Part model, mm, in its own coordinate system. Face numbers are marked on the shaded views. Round coordinates to 2 decimals unless told otherwise and drop trailing zeros. Loops run counter-clockwise (first coordinate to the right, second up) from the corner with the lowest first, then second, coordinate; pieces in that order, holes last. Notation, with made-up numbers: (-5.5, -4) -> (43.5, -4) arc R23 cw to (43.5, 7) -> close; hole circle Ø11 at (13, 15.25). An arc over 180 degrees is marked (long way). Answer as a JSON object with one key per item and string values. Group by question number.
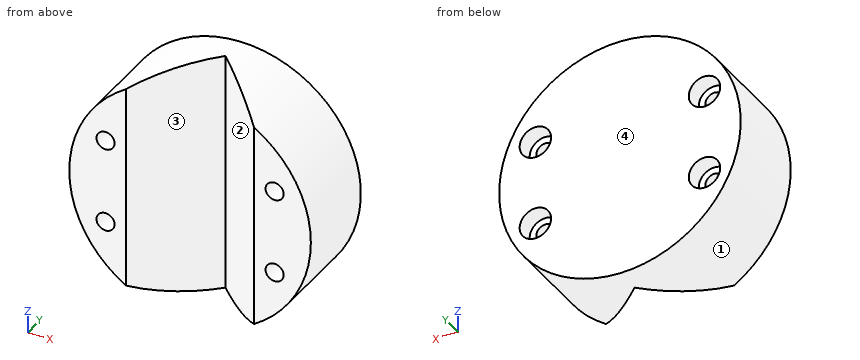
from build123d import *

# Parameters (mm, degrees)
SKETCH1_R               = 20
BOSS_EXTRUDE1_DEPTH     = 15
CUT_EXTRUDE1_DEPTH      = 25
CUT_EXTRUDE1_DEPTH_BACK = 25
CUT_EXTRUDE2_REACH      = 34.016
SKETCH3_R               = 1.5
SKETCH4_R               = 2.6
CUT_EXTRUDE3_DEPTH      = 3


with BuildPart() as part:
    # Sketch1 → Boss-Extrude1 (new body)
    with BuildSketch(Plane(origin=(0, 0, 0), x_dir=(1, 0, 0), z_dir=(0, 1, 0))):
        with Locations(Location((0, 0, 0), (0, 0, 270))):
            Circle(SKETCH1_R)
    extrude(amount=BOSS_EXTRUDE1_DEPTH)

    # Sketch2 → Cut-Extrude1 (cut, two sides: drawn at the far end of the back side and taken through both)
    with BuildSketch(Plane.XY.offset(-CUT_EXTRUDE1_DEPTH_BACK)):
        Polygon((-10.606601718, 0), (10.606601718, 0), (0, 10.606601718), align=None)
    extrude(amount=CUT_EXTRUDE1_DEPTH + CUT_EXTRUDE1_DEPTH_BACK, mode=Mode.SUBTRACT)

    # Sketch3 → Cut-Extrude2 (cut, up to next)
    with BuildSketch(Plane(origin=(0, 0, 0), x_dir=(-1, 0, 0), z_dir=(0, -1, 0)), mode=Mode.PRIVATE) as cut_extrude2_sk1:
        with Locations(Location((14, -7, 0), (0, 0, 90))):
            Circle(SKETCH3_R)
    cut_extrude2_tool1 = extrude(cut_extrude2_sk1.sketch, amount=-CUT_EXTRUDE2_REACH, mode=Mode.PRIVATE) & part.part
    # Sketch3 → Cut-Extrude2 (cut, up to next)
    with BuildSketch(Plane(origin=(0, 0, 0), x_dir=(-1, 0, 0), z_dir=(0, -1, 0)), mode=Mode.PRIVATE) as cut_extrude2_sk2:
        with Locations(Location((14, 7, 0), (0, 0, 90))):
            Circle(SKETCH3_R)
    cut_extrude2_tool2 = extrude(cut_extrude2_sk2.sketch, amount=-CUT_EXTRUDE2_REACH, mode=Mode.PRIVATE) & part.part
    # Sketch3 → Cut-Extrude2 (cut, up to next)
    with BuildSketch(Plane(origin=(0, 0, 0), x_dir=(-1, 0, 0), z_dir=(0, -1, 0)), mode=Mode.PRIVATE) as cut_extrude2_sk3:
        with Locations(Location((-14, -7, 0), (0, 0, 90))):
            Circle(SKETCH3_R)
    cut_extrude2_tool3 = extrude(cut_extrude2_sk3.sketch, amount=-CUT_EXTRUDE2_REACH, mode=Mode.PRIVATE) & part.part
    # Sketch3 → Cut-Extrude2 (cut, up to next)
    with BuildSketch(Plane(origin=(0, 0, 0), x_dir=(-1, 0, 0), z_dir=(0, -1, 0)), mode=Mode.PRIVATE) as cut_extrude2_sk4:
        with Locations(Location((-14, 7, 0), (0, 0, 90))):
            Circle(SKETCH3_R)
    cut_extrude2_tool4 = extrude(cut_extrude2_sk4.sketch, amount=-CUT_EXTRUDE2_REACH, mode=Mode.PRIVATE) & part.part
    add(cut_extrude2_tool1.solids().sort_by_distance((-14, 0, 7))[0], mode=Mode.SUBTRACT)
    add(cut_extrude2_tool2.solids().sort_by_distance((-14, 0, -7))[0], mode=Mode.SUBTRACT)
    add(cut_extrude2_tool3.solids().sort_by_distance((14, 0, 7))[0], mode=Mode.SUBTRACT)
    add(cut_extrude2_tool4.solids().sort_by_distance((14, 0, -7))[0], mode=Mode.SUBTRACT)

    # Sketch4 → Cut-Extrude3 (cut)
    with BuildSketch(Plane(origin=(0, 15, 0), x_dir=(1, 0, 0), z_dir=(0, 1, 0))):
        with Locations(Location((-14, 7, 0), (0, 0, 270))):
            Circle(SKETCH4_R)
        with Locations(Location((-14, -7, 0), (0, 0, 270))):
            Circle(SKETCH4_R)
        with Locations(Location((14, 7, 0), (0, 0, 270))):
            Circle(SKETCH4_R)
        with Locations(Location((14, -7, 0), (0, 0, 270))):
            Circle(SKETCH4_R)
    extrude(amount=-CUT_EXTRUDE3_DEPTH, mode=Mode.SUBTRACT)


solid = part.part
Item 1: Drill centre lines: line 1 (X direction, y = 7.5, z = 7) (3 decimals); line 2 (Z direction, x = -15, y = 1); line 3 (Z direction, x = 13, y = 6.75). Where is each one in solid material? Low to high.
Item 2: Band-saw the part on B-B, the plane z = -7. List the corners of the cut face in (x, y) (3 decimals).
Item 3: Band-saw the part on A-A, the plane y = 7. List the corners of the cut face in (x, z).
Item 4: Two-plate mould, pull along X, no slides. Class the marked faces 1, 2, 3 and 4: pulls with the +X half, pulls with the -X half, needs draft (parallel to the pull), parting line crosses it, or undercut.
Item 5: Drop flat-ended pins along their axis: pin 1 Ø1 at (x, y) = (3, 9) entering from -Z; pin 2 Ø2 at (y, z) = (5, -3.5) entering from +X; pin 3 Ø4 at (y, z) = (2, 2.5) entering from +X. Give the stop position or say it passes through.
Item 6: Band-saw the part on D-D, the plane z = 0. List the corners of the cut face in (x, y), plus the area to 4 significant figures.
Item 7: Band-saw the part on C-C, the plane x = -15. List the corners of the cut face in (y, z).
Entries:
{
 "1": {"line 1": "-18.735 to -15.5, -12.5 to -3.107, 3.107 to 12.5, 15.5 to 18.735", "line 2": "-13.23 to -8.12, -5.88 to 5.88, 8.12 to 13.23", "line 3": "-15.2 to -8.12, -5.88 to 5.88, 8.12 to 15.2"},
 "2": {"outline": "(-18.735, 0) -> (-15.5, 0) -> (-15.5, 12) -> (-16.6, 12) -> (-16.6, 15) -> (-18.735, 15) -> close; (-12.5, 0) -> (-10.607, 0) -> (0, 10.607) -> (10.607, 0) -> (12.5, 0) -> (12.5, 12) -> (11.4, 12) -> (11.4, 15) -> (-11.4, 15) -> (-11.4, 12) -> (-12.5, 12) -> close; (15.5, 0) -> (18.735, 0) -> (18.735, 15) -> (16.6, 15) -> (16.6, 12) -> (15.5, 12) -> close"},
 "3": {"outline": "(-3.61, -19.67) -> (-3.61, 19.67) arc R20 ccw to start; (3.61, -19.67) arc R20 ccw to (3.61, 19.67) -> close; hole circle Ø3 at (-14, -7); hole circle Ø3 at (-14, 7); hole circle Ø3 at (14, -7); hole circle Ø3 at (14, 7)"},
 "4": {"face 1": "parting line crosses it", "face 2": "undercut", "face 3": "undercut", "face 4": "needs draft"},
 "5": {"pin 1": "z = -19.84", "pin 2": "x = 19.84", "pin 3": "x = 19.99"},
 "6": {"outline": "(-20, 0) -> (-10.61, 0) -> (0, 10.61) -> (10.61, 0) -> (20, 0) -> (20, 15) -> (-20, 15) -> close", "area": "487.5 mm²"},
 "7": {"outline": "(0, -13.23) -> (15, -13.23) -> (15, -9.4) -> (12, -9.4) -> (12, -8.12) -> (0, -8.12) -> close; (0, -5.88) -> (12, -5.88) -> (12, -4.6) -> (15, -4.6) -> (15, 4.6) -> (12, 4.6) -> (12, 5.88) -> (0, 5.88) -> close; (0, 8.12) -> (12, 8.12) -> (12, 9.4) -> (15, 9.4) -> (15, 13.23) -> (0, 13.23) -> close"}
}
